```python
from build123d import *

# Parameters (mm, degrees)
F3_DEPTH = 1.6
F4_SIZE2 = 0.8660254038
F4_SIZE  = 0.5
F5_SIZE  = 0.3
F6_R     = 0.1


with BuildPart() as f1:
    # F0 (on Front) → F1 (revolve)
    with BuildSketch(Plane.XZ):
        Polygon((2.75, 0), (0, 0), (0, -11), (1.5, -11), (1.5, -3), (2.75, -3), align=None)
    revolve(axis=Axis((0, 0, -5.5), (0, 0, 1)))

    # F2 (on face) → F3 (cut)
    with BuildSketch(Plane.XY):
        Polygon((0.7216878365, 1.25), (-0.7216878365, 1.25), (-1.443375673, 0), (-0.7216878365, -1.25), (0.7216878365, -1.25), (1.443375673, 0), align=None)
    extrude(amount=-F3_DEPTH, mode=Mode.SUBTRACT)

    # F4
    f4_edges = [f1.edges().sort_by_distance(p)[0] for p in [
        (0, 1.25, -1.6),
        (-1.082532, 0.625, -1.6),
        (-1.082532, -0.625, -1.6),
        (0, -1.25, -1.6),
        (1.082532, -0.625, -1.6),
        (1.082532, 0.625, -1.6),
    ]]
    chamfer(f4_edges, length=F4_SIZE, length2=F4_SIZE2)

    # F5
    f5_edges = [f1.edges().sort_by_distance(p)[0] for p in [
        (-2.75, 0, 0),
        (-1.5, 0, -11),
    ]]
    chamfer(f5_edges, length=F5_SIZE)

    # F6
    f6_edges = [f1.edges().sort_by_distance(p)[0] for p in [
        (-2.75, 0, -3),
    ]]
    fillet(f6_edges, radius=F6_R)


with BuildPart() as f7_1:
    # F7: copy of F1
    add(f1.part)


solid = f1.part
```
Geometry check sheet. Reference: the model listing, model coordinates, mm. A direction names the side the tool comes from. Coordinates: 2 decimals unless noted, no trailing zeros. Order: outer loops, then holes, each group sorted by start corner. A loop starts at its lowest first (then second) coordinate and runs counter-clockwise, first axis right, second up. Notation, with made-up numbers: M -12.75,-30.75 L 2.25,-30.75 A25 ccw 2.25,-5.75 Z; hole C -11.75,-30 d8. An arc over 180 degrees is marked long. One line per question, with ' | ' between items. Start each with the question number.
Item 1: Draft check along X on faces 1 (the flat face through (1.1, -1.1, 0)), 2 (the flat face through (1.08, -0.63, -0.54)), 3 (the cylindrical face through (-1.5, 0.07, -6.8)). Enter one of: pulls with the +X half, pulls with the -X half, needs draft (parallel to the pull), parting line crosses it, or undercut.
Item 2: Gauge pin test, flat ends, axial feed: pin 1 (1.5 mm diameter, centred on y = 1, z = -5, fed in from -X); pin 2 (1 mm diameter, centred on x = 0, z = -4, fed in from -Y). Record the tip position at first contact, or that the pin passes through.
Item 3: Material ranges on L1, parallel to Z at x = 1.9, y = 1.45; L2, parallel to X at y = 0.05, z = -3.5; L3, parallel to Y at x = 0.7, z = -1, recorded low to high. Write a range as [from, to].
Item 4: Cross-section at B-B on z = -7.25. Enter the section's corners in (x, y).
Item 5: Cross-section at A-A on x = 0. Enter the section's corners in (y, z), then the cut area to 3 significant figures.
Item 6: Set-up check for faces 4 (the flat face through (0, -0.9, -1.3)), 5 (the flat face through (0, -2, -3)), 6 (the cylindrical face through (-0.596, -2.685, -1.582)): record each of +Z, -Z, +X, -X, +Y, -Y from which the full face is reachable in a straight line by a thin tool's end or side.
Findings:
1) face 1: needs draft | face 2: undercut | face 3: parting line crosses it
2) pin 1: stops at x = -1.48 | pin 2: stops at y = -1.5
3) L1: z = [-3, 0] | L2: x = [-1.5, 1.5] | L3: y = [-2.66, -1.25], [1.25, 2.66]
4) outline: C 0,0 d3
5) outline: M -2.75,-2.9 A0.1 ccw -2.65,-3 L -1.5,-3 L -1.5,-10.7 L -1.2,-11 L 1.2,-11 L 1.5,-10.7 L 1.5,-3 L 2.65,-3 A0.1 ccw 2.75,-2.9 L 2.75,-0.3 L 2.45,0 L 1.25,0 L 1.25,-1.1 L 0.38,-1.6 L -0.38,-1.6 L -1.25,-1.1 L -1.25,0 L -2.45,0 L -2.75,-0.3 Z | area: 36.7 mm²
6) face 4: +Z | face 5: -Z | face 6: +Z, -Z
